Input: part model. Units: mm. Frame: model coordinates. A direction names the side the tool comes from. Coordinates: 2 decimals unless noted, no trailing zeros. Write each loop counter-clockwise with the first axis right and the second up, starting at its lowest first coordinate (ties: lowest second). Pieces come first, ordered by that corner, then holes.
from build123d import *

# Parameters (mm, degrees)
F0_W          = 101.6
F0_H          = 101.6
F1_DEPTH      = 609.6
F2_R          = 19.05
F3_DEPTH      = 406.4
F3_DEPTH_BACK = 508
F4_W          = 0.79375
F4_H          = 609.6
F5_DEPTH      = 25.4
F6_R          = 25.4
F7_R          = 25.4


with BuildPart() as f1:
    # F0 (on Front) → F1 (new body)
    with BuildSketch(Plane.XZ):
        Polygon((-103.1875, -22.225), (-103.1875, 1.5875), (-77.7875, 1.5875), (-77.7875, 3.175), (-104.775, 3.175), (-104.775, -22.225), align=None)
        Polygon((-77.7875, 1.5875), (-103.1875, 1.5875), (-103.1875, -22.225), (-103.1875, -79.375), (-103.1875, -103.1875), (-77.7875, -103.1875), (-23.8125, -103.1875), (1.5875, -103.1875), (1.5875, -79.375), (1.5875, -22.225), (1.5875, 1.5875), (-23.8125, 1.5875), align=None)
        with Locations((-50.8, -50.8)):
            Rectangle(F0_W, F0_H, mode=Mode.SUBTRACT)
        Polygon((-103.1875, -103.1875), (-103.1875, -79.375), (-104.775, -79.375), (-104.775, -104.775), (-77.7875, -104.775), (-77.7875, -103.1875), align=None)
        Polygon((3.175, -79.375), (1.5875, -79.375), (1.5875, -103.1875), (-23.8125, -103.1875), (-23.8125, -104.775), (3.175, -104.775), align=None)
        Polygon((-23.8125, 3.175), (-23.8125, 1.5875), (1.5875, 1.5875), (1.5875, -22.225), (3.175, -22.225), (3.175, 3.175), align=None)
    extrude(amount=F1_DEPTH)

    # F2 (on face) → F3 (join, two sides)
    with BuildSketch(Plane.YZ.offset(1.5875)) as f3_sk:
        with Locations((-304.8, -50.8)):
            Circle(F2_R)
    extrude(amount=F3_DEPTH)
    extrude(f3_sk.sketch, amount=-F3_DEPTH_BACK)

    # F4 (on face) → F5 (join)
    with BuildSketch(Plane(origin=(0, 0, -103.1875), x_dir=(1, 0, 0), z_dir=(0, 0, -1))):
        with Locations((-50.403125, 304.8)):
            Rectangle(F4_W, F4_H)
        with Locations((-51.196875, 304.8)):
            Rectangle(F4_W, F4_H)
    extrude(amount=F5_DEPTH)

    # F6
    f6_edges = [f1.edges().sort_by_distance(p)[0] for p in [
        (-50.8, 0, -128.5875),
    ]]
    fillet(f6_edges, radius=F6_R)

    # F7
    f7_edges = [f1.edges().sort_by_distance(p)[0] for p in [
        (-50.8, -609.6, -128.5875),
    ]]
    fillet(f7_edges, radius=F7_R)


solid = f1.part
Item 1: Material intervals for line 1 (X direction, y = -556, z = -21) (3 decimals); line 2 (X direction, y = -553.5, z = -74), sorted ascending.
Item 2: Section query B-B, the plane z = -50.8. Return loops of the section in (x, y).
Item 3: Section query D-D, the plane x = 163.5. Return loops of the section in (y, z).
Item 4: Access query for faces 1 (the face through (-52, -301, -101.6)), 2 (the face through (-37, -301, -103.188)), 3 (the face through (-91, -301, -104.775)), 4 (the face through (1.588, -301, -70)). Directions: +Z, -Z, +X, -X, +Y, -Y. A direction counts if a zero-diameter tool reaches every point of the face in a straight line with its end or side. Return the directions, or none.
Item 5: Section query A-A, the plane y = -159. Return loops of the section in (x, z) (1 decimal).
Item 6: Pin query (flat end, axial travel): pin 1 Ø3 at (y, z) = (-80, -41.5) entering from -X; pin 2 Ø17 at (y, z) = (-420, -38) entering from +X; pin 3 Ø6 at (x, z) = (-82, -71) entering from +Y. Return the tip coordinate at first contact, or that it passes through.
Item 7: Section query C-C, the plane y = -304.8. State how many separate pieces and enclosed holes the cut face has, then the cut area to 3 significant figures.
Item 8: Pull-direction query (Z, two-part tool) for faces 5 (the face through (0, -301, -29)), 6 (the face through (407.987, -305, -51)), 7 (the face through (-91, -301, 3.175)), 8 (the face through (-11, -301, -104.775)); classes: released by +Z, released by -Z, zero draft, split by the parting line, or undercut.
The answers:
1. line 1: x = -104.775 to -101.6, 0 to 3.175
1. line 2: x = -103.19 to -101.6, 0 to 1.59
2. outline: (-506.41, -323.85) - (-103.19, -323.85) - (-103.19, -609.6) - (-101.6, -609.6) - (-101.6, -323.85) - (0, -323.85) - (0, -609.6) - (1.59, -609.6) - (1.59, -323.85) - (407.99, -323.85) - (407.99, -285.75) - (1.59, -285.75) - (1.59, 0) - (0, 0) - (0, -285.75) - (-101.6, -285.75) - (-101.6, 0) - (-103.19, 0) - (-103.19, -285.75) - (-506.41, -285.75) - close
3. outline: circle Ø38.1 at (-304.8, -50.8)
4. face 1: +Y, -Y
4. face 2: -Z, +Y, -Y
4. face 3: -Z, -X, +Y, -Y
4. face 4: +X
5. outline: (-104.8, -104.8) - (-77.8, -104.8) - (-77.8, -103.2) - (-51.6, -103.2) - (-51.6, -128.6) - (-50, -128.6) - (-50, -103.2) - (-23.8, -103.2) - (-23.8, -104.8) - (3.2, -104.8) - (3.2, -79.4) - (1.6, -79.4) - (1.6, -22.2) - (3.2, -22.2) - (3.2, 3.2) - (-23.8, 3.2) - (-23.8, 1.6) - (-77.8, 1.6) - (-77.8, 3.2) - (-104.8, 3.2) - (-104.8, -22.2) - (-103.2, -22.2) - (-103.2, -79.4) - (-104.8, -79.4) - close; hole (-101.6, -101.6) - (0, -101.6) - (0, 0) - (-101.6, 0) - close
6. pin 1: stops at x = -103.19
6. pin 2: stops at x = 1.59
6. pin 3: stops at y = -296.61
7. separate pieces: 1
7. enclosed holes: 2
7. area: 35,700 mm2
8. face 5: undercut
8. face 6: zero draft
8. face 7: released by +Z
8. face 8: released by -Z
